Verification items for the finished model (mm, model axes). Face numbers are marked on the shaded views. Coordinates: 2 decimals unless noted, no trailing zeros. Order: outer loops, then holes, each group sorted by start corner. A loop starts at its lowest first (then second) coordinate and runs counter-clockwise, first axis right, second up. Notation, with made-up numbers: M 22,77 L 28,77 A20 cw 28,92 Z; hole C -6,24.5 d3. An arc over 180 degrees is marked long. Answer as a JSON object with one key per item and string values. Group by question number.
(1) Material ranges on line 1 (Z direction, x = 22, y = 10.5), recorded low to high.
(2) Gauge pin test, flat ends, axial feed: pin 1 Ø6.5 at (x, y) = (18, 15.5) entering from +Z; pin 2 Ø0.8 at (x, z) = (1, 10) entering from -Y. Record the tip position at first contact, or that the pin passes through.
(3) Mould release check, pull along Y, two halves, no side actions. Record for the marked faces 1, 2, 3 and 4: released by +Y, released by -Y, zero draft, split by the parting line, or undercut.
(4) Cross-section at A-A (x = 17). Enter the section's corners in (y, z).
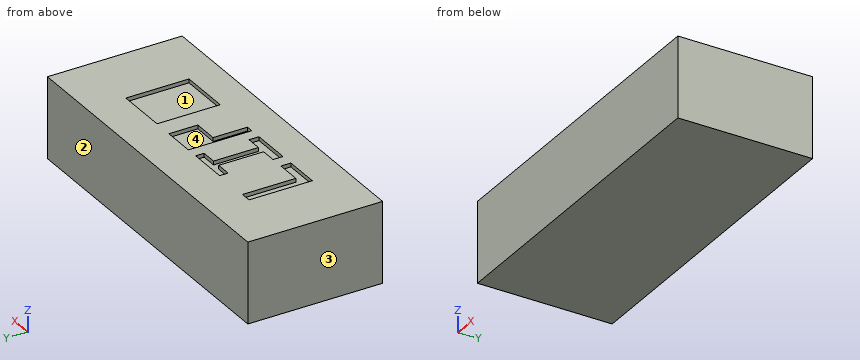
from build123d import *

# Parameters (mm, degrees)
SKETCH1_W           = 86
SKETCH1_H           = 21
BOSS_EXTRUDE1_DEPTH = 35
SKETCH2_W           = 13.394867866
SKETCH2_H           = 16.41192305
CUT_EXTRUDE1_DEPTH  = 1


with BuildPart() as part:
    # Sketch1 → Boss-Extrude1 (new body)
    with BuildSketch(Plane(origin=(0, 0, 0), x_dir=(1, 0, 0), z_dir=(0, 1, 0))):
        Rectangle(SKETCH1_W, SKETCH1_H)
    extrude(amount=BOSS_EXTRUDE1_DEPTH)

    # Sketch2 → Cut-Extrude1 (cut)
    with BuildSketch(Plane.XY.offset(10.5)):
        Polygon((-27.062922658, 25.043511527), (-27.062922658, 8.589083039), (-17.841816761, 8.589083039), (-17.841816761, 11.184244579), (-24.246896306, 11.184244579), (-24.246896306, 25.043511527), align=None)
        Polygon((-14.472064369, 25.043511527), (-4.155267693, 25.043511527), (-4.155267693, 22.842768469), (-8.207777961, 22.842768469), (-8.207777961, 11.184244579), (-4.155267693, 11.184244579), (-4.155267693, 8.589083039), (-14.472064369, 8.589083039), (-14.472064369, 11.184244579), (-10.419554101, 11.184244579), (-10.419554101, 22.842768469), (-14.472064369, 22.842768469), align=None)
        Polygon((-1.057635761, 25.043511527), (-1.057635761, 8.589083039), (0.791487413, 8.589083039), (0.791487413, 17.514312266), (7.331069367, 17.514312266), (7.331069367, 25.043511527), align=None)
        with Locations((19.169967733, 16.795044564)):
            Rectangle(SKETCH2_W, SKETCH2_H)
    extrude(amount=-CUT_EXTRUDE1_DEPTH, mode=Mode.SUBTRACT)


solid = part.part
Taken from the geometry:
{
 "1": {"line 1": "z = -10.5 to 9.5"},
 "2": {"pin 1": "stops at z = 9.5", "pin 2": "stops at y = 0"},
 "3": {"face 1": "undercut", "face 2": "released by +Y", "face 3": "zero draft", "face 4": "undercut"},
 "4": {"outline": "M 0,-10.5 L 35,-10.5 L 35,10.5 L 25,10.5 L 25,9.5 L 8.59,9.5 L 8.59,10.5 L 0,10.5 Z"}
}
